from build123d import *

# Parameters (mm, degrees)
BOSS_EXTRUDE1_DEPTH = 49.9745
SKETCH2_R           = 2.0193
CUT_EXTRUDE1_DEPTH  = 19.05
SKETCH3_R           = 11.064818238
SKETCH3_R_2         = 5.125
CUT_EXTRUDE2_DEPTH  = 7.112


with BuildPart() as part:
    # Sketch1 → Boss-Extrude1 (new, symmetric)
    with BuildSketch(Plane.XY):
        Polygon((4.7625, 2.749630657), (0, 5.499261314), (-4.7625, 2.749630657), (-4.7625, -2.749630657), (0, -5.499261314), (4.7625, -2.749630657), align=None)
    extrude(amount=BOSS_EXTRUDE1_DEPTH, both=True)

    # Sketch2 → Cut-Extrude1 (cut)
    with BuildSketch(Plane(origin=(0, 0, -49.9745), x_dir=(-1, 0, 0), z_dir=(0, 0, -1))):
        Circle(SKETCH2_R)
    cut_extrude1 = extrude(amount=-CUT_EXTRUDE1_DEPTH, mode=Mode.SUBTRACT)

    # Mirror1: Cut-Extrude1 across plane
    add(cut_extrude1.mirror(Plane.XY), mode=Mode.SUBTRACT)

    # Sketch3 → Cut-Extrude2 (cut)
    with BuildSketch(Plane(origin=(0, 0, -49.9745), x_dir=(-1, 0, 0), z_dir=(0, 0, -1))):
        Circle(SKETCH3_R)
        Circle(SKETCH3_R_2, mode=Mode.SUBTRACT)
    cut_extrude2 = extrude(amount=-CUT_EXTRUDE2_DEPTH, mode=Mode.SUBTRACT)

    # Mirror2: Cut-Extrude2 across plane
    add(cut_extrude2.mirror(Plane.XY), mode=Mode.SUBTRACT)


solid = part.part
Here's how the part is built. I have some questions about the finished solid (model axes, mm). A direction names the side the tool comes from. Coordinates: 2 decimals unless noted, no trailing zeros. Write each loop counter-clockwise with the first axis right and the second up, starting at its lowest first coordinate (ties: lowest second). Pieces come first, ordered by that corner, then holes.
1) Which directions (+Z, -Z, +X, -X, +Y, -Y) give clear straight access to the entire face, cutting with the end or side of a thin tool? Please do faces 1 (the face through (-1.926, 0.607, 40.583)), 2 (the face through (0, 0, -30.924)), 3 (the face through (2.41, 4.11, 0.7)).
Filled in:
face 1: +Z
face 2: -Z
face 3: +Z, -Z, +X, +Y
2) If we section it at C-C (x = 3): List the corners of the cut face in (y, z) for me, plus the area to 3 significant figures.
Filled in:
outline: (-3.77, -49.97) - (3.77, -49.97) - (3.77, 49.97) - (-3.77, 49.97) - close
area: 753 mm2
3) If we section it at B-B (z = -29.5): List the corners of the cut face in (x, y) for me.
Filled in:
outline: (-4.76, -2.75) - (0, -5.5) - (4.76, -2.75) - (4.76, 2.75) - (0, 5.5) - (-4.76, 2.75) - close
4) If we section it at D-D (y = -4): List the corners of the cut face in (x, z) for me, plus the area to 3 significant figures.
Filled in:
outline: (-2.6, -49.97) - (2.6, -49.97) - (2.6, 49.97) - (-2.6, 49.97) - close
area: 519 mm2
5) Thinking about a two-plate mould opening in Y: for faces 4 (the face through (0, 0, 30.924)), 5 (the face through (-4.762, 0, 1)), 6 (the face through (2.348, -4.144, 0.7)), which applies, +Y half, -Y half, draft (parallel to the pull), parting line (faces both ways), or undercut?
Filled in:
face 4: undercut
face 5: draft
face 6: -Y half
6) I'm going to push flat-ended pins straight in: pin 1 (0.8 mm diameter, centred on x = 4.5, y = 3, fed in from +Z); pin 2 (3 mm diameter, centred on y = 4.5, z = 36.5, fed in from +X); pin 3 (0.5 mm diameter, centred on x = 0, y = -5.5, fed in from -Z); pin 4 (1.2 mm diameter, centred on x = -0.5, y = 1, fed in from +Z). Where does each tip first touch, or does it pass through?
Filled in:
pin 1: stops at z = 49.97
pin 2: stops at x = 4.33
pin 3: stops at z = -42.86
pin 4: stops at z = 30.92
7) If we section it at A-A (y = 0): List the corners of the cut face in (x, z) for me, plus the area to 3 significant figures.
Filled in:
outline: (-4.76, -49.97) - (-2.02, -49.97) - (-2.02, -30.92) - (2.02, -30.92) - (2.02, -49.97) - (4.76, -49.97) - (4.76, 49.97) - (2.02, 49.97) - (2.02, 30.92) - (-2.02, 30.92) - (-2.02, 49.97) - (-4.76, 49.97) - close
area: 798 mm2
8) If I drill on line 1 (Y direction, x = 0, z = -40.25); line 2 (Y direction, x = 0, z = -45.75) (3 decimals); line 3 (X direction, y = -0.75, z = 39), over which ranges is the centre line in solid material (lowest first)?
Filled in:
line 1: y = -5.5 to -2.02, 2.02 to 5.5
line 2: y = -5.125 to -2.019, 2.019 to 5.125
line 3: x = -4.76 to -1.87, 1.87 to 4.76
